```python
from build123d import *

# Parameters (mm, degrees)
F0_W     = 104.0173918009
F0_H     = 5
F1_DEPTH = 2
F2_DEPTH = 16
F3_SIZE2 = 1.819841
F3_SIZE  = 4.99999


# Not quite as in the source:
# - a fillet or chamfer is up to 0.001 mm smaller than in the source, because OpenCascade refuses the exact size


with BuildPart() as f1:
    # F0 (on Top) → F1 (new body)
    with BuildSketch(Plane.XY):
        Polygon((-72.627124867, 48.6539505273), (-75.627124867, 48.6539505273), (-75.627124867, -74.8460494727), (-72.627124867, -74.8460494727), (-14.627124867, -74.8460494727), (-14.3716531694, -74.8460494727), (43.372875133, -74.8460494727), (46.372875133, -74.8460494727), (46.372875133, 48.6539505273), (43.372875133, 48.6539505273), (-14.3716531694, 48.6539505273), (-14.627124867, 48.6539505273), (-14.8716531694, 48.6539505273), align=None)
        with Locations((-15.4112055898, 18.7856731331)):
            Rectangle(F0_W, F0_H, mode=Mode.SUBTRACT)
        with Locations((-15.4112055898, 18.7856731331)):
            Rectangle(F0_W, F0_H)
    extrude(amount=-F1_DEPTH)

    # F0 (on Top) → F2 (join)
    with BuildSketch(Plane.XY):
        with Locations((-15.4112055898, 18.7856731331)):
            Rectangle(F0_W, F0_H)
    extrude(amount=F2_DEPTH)

    # F3 (size 5 and 1.8198511713 in the source; OpenCascade refuses exactly that, so slightly less here)
    f3_edges = [f1.edges().sort_by_distance(p)[0] for p in [
        (-15.411206, 16.285673, 16),
    ]]
    f3_side = f1.faces().sort_by_distance((-15.411206, 18.785673, 16))[0]
    chamfer(f3_edges, length=F3_SIZE, length2=F3_SIZE2, reference=f3_side)


solid = f1.part
```
Can you work these out from the model? Positions are in its coordinate system, mm. A direction names the side the tool comes from. Coordinates: 2 decimals unless noted, no trailing zeros. Write each loop counter-clockwise with the first axis right and the second up, starting at its lowest first coordinate (ties: lowest second). Pieces come first, ordered by that corner, then holes. Notation, with made-up numbers: M 78.25,83 L 108.25,83 A21 ccw 108.25,102 Z; hole C 86,82 d5. An arc over 180 degrees is marked long. Answer as CSV lines item,"result".
Item 1: On a 3-axis mill with a long thin cutter (end or side, diameter ignored), from which of +Z, -Z, +X, -X, +Y, -Y can I reach the whole of each face in a straight line? I mean faces 1 (the flat face through (36.597, 19, 8)), 2 (the flat face through (-67.42, 19, 8)), 3 (the flat face through (-16, 21.286, 8)), 4 (the flat face through (-16, 16.286, 7)), 5 (the flat face through (-15, -12, -2)). Say none if no direction works.
Geometry results:
face 1,"+Z, +X, +Y, -Y"
face 2,"+Z, -X, +Y, -Y"
face 3,"+Z, +X, -X, +Y"
face 4,"+Z, +X, -X, -Y"
face 5,"-Z, +X, -X, +Y, -Y"
Item 2: Imagine slicing it at C-C on z = 1.75. List the corners of the cut face in (x, y) for me, plus the area to 3 significant figures.
Geometry results:
outline,"M -67.42,16.29 L 36.6,16.29 L 36.6,21.29 L -67.42,21.29 Z"
area,"520 mm2"
Item 3: Imagine slicing it at B-B on y = -5. List the corners of the cut face in (x, z) for me.
Geometry results:
outline,"M -75.63,-2 L 46.37,-2 L 46.37,0 L -75.63,0 Z"
Item 4: I'm going to push flat-ended pins straight in: P1, Ø3, axis at x = -55, z = 10.5, coming from the +Y side; P2, Ø2.5, axis at y = 19.5, z = 10.5, coming from the +X side; P3, Ø7, axis at x = -15, z = 9, coming from the -Y side. Where does each tip first touch, or does it pass through?
Geometry results:
P1,"stops at y = 21.29"
P2,"stops at x = 36.6"
P3,"stops at y = 16.29"
Item 5: Please list where these lines run through material, in increasing order: line 1 along Y through (x, z) = (-16, 9); line 2 along Z through (x, y) = (26, -30).
Geometry results:
line 1,"y = 16.29 to 21.29"
line 2,"z = -2 to 0"
